```python
from build123d import *

# Parameters (mm, degrees)
F1_DEPTH = 31.4452
F3_R     = 1.686467
F4_DEPTH = 25.4
F3_R_2   = 1.420474
F5_DEPTH = 25.4


with BuildPart() as f1:
    # F0 (on Front) → F1 (new body)
    with BuildSketch(Plane.XZ):
        Polygon((-8.363467, 10.70378), (-25.210224, 10.70378), (-25.210224, -10.70378), (25.210224, -10.70378), (25.210224, 10.70378), (10.432723, 10.70378), (10.432723, 18.035768), (-8.363467, 18.035768), align=None)
    extrude(amount=-F1_DEPTH)

    # F3 (on face) → F4 (cut)
    with BuildSketch(Plane(origin=(0, 0, -10.70378), x_dir=(1, 0, 0), z_dir=(0, 0, -1))):
        with Locations((20.485872, -14.341232)):
            Circle(F3_R)
    extrude(amount=-F4_DEPTH, mode=Mode.SUBTRACT)

    # F3 (on face) → F5 (cut)
    with BuildSketch(Plane(origin=(0, 0, -10.70378), x_dir=(1, 0, 0), z_dir=(0, 0, -1))):
        with Locations((20.874409, -22.897052)):
            Circle(F3_R_2)
    extrude(amount=-F5_DEPTH, mode=Mode.SUBTRACT)


solid = f1.part
```
CAD build for the part. Positions are in the model's coordinates, mm. A direction names the side the tool comes from. Round coordinates to 2 decimals unless told otherwise and drop trailing zeros. Write each loop counter-clockwise with the first axis right and the second up, starting at its lowest first coordinate (ties: lowest second). Pieces come first, ordered by that corner, then holes. Notation, with made-up numbers: (87, 80.5) -> (100, 80.5) arc R14 cw to (100, 90.5) -> close; hole circle Ø6 at (45.25, 67). An arc over 180 degrees is marked (long way). Answer in a Markdown table with one row per item. Add a question column.
Item 1: Saw through at B-B, the plane y = 8. Write the cut outline in (x, z).
Item 2: Mould opens along X. For faces 1 (the face through (19.827, 21.937, -0.15)), 2 (the face through (25.21, 16, 0)), 3 (the face through (1, 16, 18.036)) say: pulls with the +X half, pulls with the -X half, needs draft (parallel to the pull), parting line crosses it, or undercut.
Item 3: Which spindle directions (+Z, -Z, +X, -X, +Y, -Y) get a long thin tool onto all of the face, cutting with end or side? Do faces 4 (the face through (0, 0, 1)), 5 (the face through (-17, 16, 10.704)), 6 (the face through (18, 16, 10.704)). Say none if no direction does.
Item 4: Saw through at D-D, the plane x = -17.5. Write the cut outline in (y, z).
Item 5: Drill centre lines: line 1 (Z direction, x = 21, y = 29); line 2 (X direction, y = 15, z = -6.25); line 3 (X direction, y = 22, z = 14.5). Where is each one in solid material? Low to high. Write a range as from..to.
Item 6: Saw through at C-C, the plane z = 12.25. Write the cut outline in (x, y).
Item 7: Drop flat-ended pins along their axis: pin 1 Ø12 at (x, y) = (17, 8) entering from +Z; pin 2 Ø2 at (x, y) = (20.49, 14.34) entering from +Z; pin 3 Ø6 at (y, z) = (14, 16) entering from -X. Give the stop position or say it passes through.
Item 8: Saw through at A-A, the plane x = 20. Write the cut outline in (y, z).
Findings below:
| question | item | result |
|---|---|---|
| 1 | outline | (-25.21, -10.7) -> (25.21, -10.7) -> (25.21, 10.7) -> (10.43, 10.7) -> (10.43, 18.04) -> (-8.36, 18.04) -> (-8.36, 10.7) -> (-25.21, 10.7) -> close |
| 2 | face 1 | undercut |
| 2 | face 2 | pulls with the +X half |
| 2 | face 3 | needs draft |
| 3 | face 4 | +Z, -Z, +X, -X, -Y |
| 3 | face 5 | +Z, -X, +Y, -Y |
| 3 | face 6 | +Z, +X, +Y, -Y |
| 4 | outline | (0, -10.7) -> (31.45, -10.7) -> (31.45, 10.7) -> (0, 10.7) -> close |
| 5 | line 1 | z = -10.7..10.7 |
| 5 | line 2 | x = -25.21..18.93, 22.04..25.21 |
| 5 | line 3 | x = -8.36..10.43 |
| 6 | outline | (-8.36, 0) -> (10.43, 0) -> (10.43, 31.45) -> (-8.36, 31.45) -> close |
| 7 | pin 1 | stops at z = 10.7 |
| 7 | pin 2 | passes through |
| 7 | pin 3 | stops at x = -8.36 |
| 8 | outline | (0, -10.7) -> (12.73, -10.7) -> (12.73, 10.7) -> (0, 10.7) -> close; (15.96, -10.7) -> (21.78, -10.7) -> (21.78, 10.7) -> (15.96, 10.7) -> close; (24.02, -10.7) -> (31.45, -10.7) -> (31.45, 10.7) -> (24.02, 10.7) -> close |
